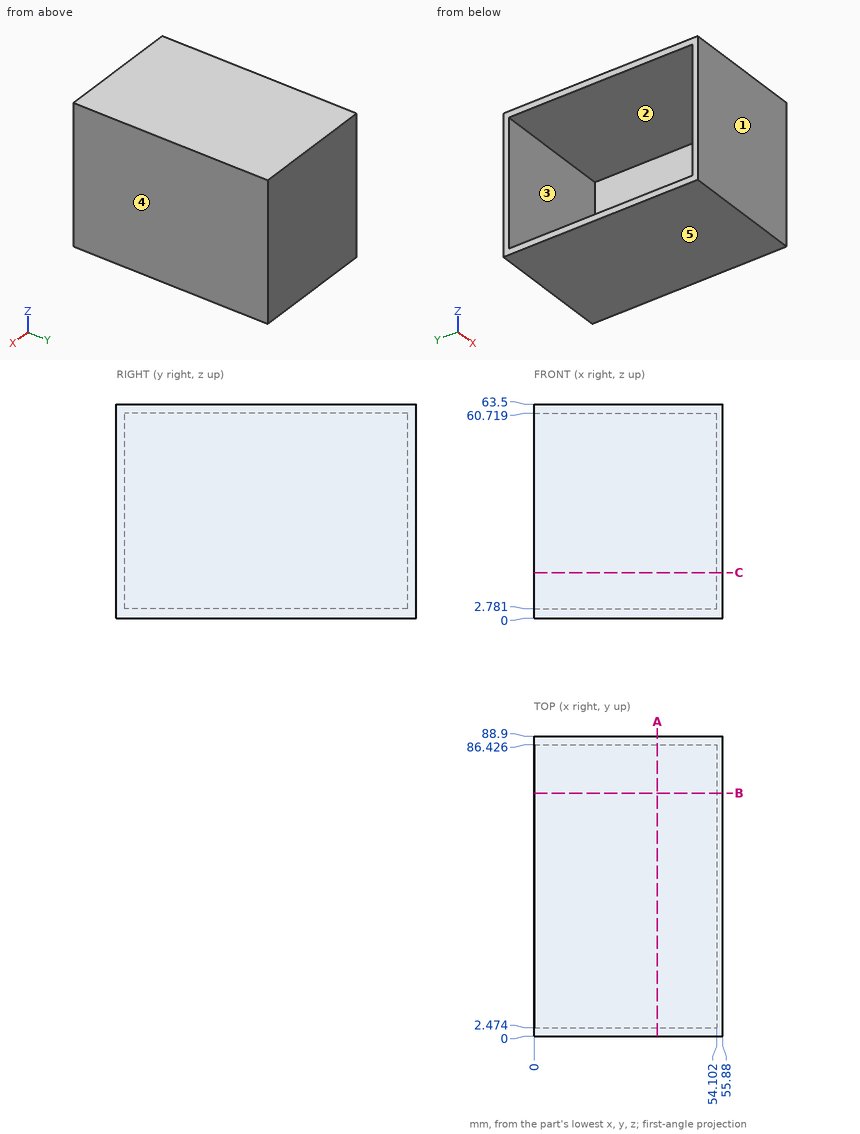
The drawing under review shows one solid part. Ordinate dimensions are in mm from its lowest x, y, z. A direction names the side the tool comes from. Give positions to 0.01 mm unless a question says otherwise; leave off trailing zeros. Order: outer loops, then holes, each group sorted by start corner. A loop starts at its lowest first (then second) coordinate and runs counter-clockwise, first axis right, second up. Notation, with made-up numbers: (47, 17) - (57, 17) arc R14 cw to (57, 30) - close; hole circle Ø6 at (-23.5, -5). An arc over 180 degrees is marked (long way). Answer as a JSON object with one key per item and string values. Group by question number.
Item 1: Take a section at C-C on z = 13.5. Give the boundary of the cut face in (x, y), and give its area (3 significant figures).
Item 2: Wall thickness on line 1 along Y through (x, z) = (43.5, 21.5); line 2 along Z through (x, y) = (19.5, 46.5); line 3 along X through (y, z) = (53.5, 57): over which ranges is each line inside the solid? List them lowest first.
Item 3: Take a section at B-B on y = 72. Give the boundary of the cut face in (x, z), and give its area (3 significant figures).
Item 4: Clearance check with flat-ended pins moving along their axes: pin 1 Ø2 at (x, z) = (35, 47.5) entering from -Y; pin 2 Ø10 at (y, z) = (61.5, 47) entering from -X. State where each tip first meets the part, or that it passes through.
Item 5: Take a section at A-A on x = 36.5. Give the boundary of the cut face in (y, z).
Item 6: Machinability: for the marked faces 1 and 2, which of the approach directions +Z, -Z, +X, -X, +Y, -Y give a long, thin tool a straight path to every point of the face, cutting with its end or side? Answer none if there is none.
Item 7: Draft analysis for pull direction Z (two halves, no side actions). For the marked faces 3, 4 and 5, state which applies: pulls with the +Z half, pulls with the -Z half, needs draft (parallel to the pull), parting line crosses it, or undercut.
Reported:
{
 "1": {"outline": "(0, 0) - (55.88, 0) - (55.88, 88.9) - (0, 88.9) - (0, 86.43) - (54.1, 86.43) - (54.1, 2.47) - (0, 2.47) - close", "area": "426 mm^2"},
 "2": {"line 1": "0 to 2.47, 86.43 to 88.9", "line 2": "0 to 2.78, 60.72 to 63.5", "line 3": "54.1 to 55.88"},
 "3": {"outline": "(0, 0) - (55.88, 0) - (55.88, 63.5) - (0, 63.5) - (0, 60.72) - (54.1, 60.72) - (54.1, 2.78) - (0, 2.78) - close", "area": "414 mm^2"},
 "4": {"pin 1": "y = 0", "pin 2": "x = 54.1"},
 "5": {"outline": "(0, 0) - (88.9, 0) - (88.9, 63.5) - (0, 63.5) - close; hole (2.47, 2.78) - (86.43, 2.78) - (86.43, 60.72) - (2.47, 60.72) - close"},
 "6": {"face 1": "+Z, -Z, +X, -X, -Y", "face 2": "-X"},
 "7": {"face 3": "undercut", "face 4": "needs draft", "face 5": "pulls with the -Z half"}
}
